from build123d import *

# Parameters (mm, degrees)
BOSS_EXTRUDE3_DEPTH = 30
CUT_EXTRUDE1_DEPTH  = 36.393360959
SKETCH12_W          = 4
SKETCH12_H          = 13
BOSS_EXTRUDE4_DEPTH = 30
BOSS_EXTRUDE9_REACH = 63.617
CUT_EXTRUDE3_DEPTH  = 55.655521025
CUT_EXTRUDE4_REACH  = 52.517


with BuildPart() as part:
    # Sketch7 → Boss-Extrude3 (new body)
    with BuildSketch(Plane.XY):
        Polygon((-1.7, -2), (-1.7, -15), (-5.7, -15), (-5.7, -2), (-9, -2), (-9, -15), (-13, -15), (-13, 1.250897452), align=None)
    extrude(amount=BOSS_EXTRUDE3_DEPTH)

    # Sketch11 → Cut-Extrude1 (cut, through all)
    with BuildSketch(Plane.ZY.offset(13)):
        Polygon((0, 1.250897452), (7.323081285, -15), (0, -15), align=None)
    extrude(amount=-CUT_EXTRUDE1_DEPTH, mode=Mode.SUBTRACT)

    # Sketch12 → Boss-Extrude4 (add, along a direction that is not the sketch's normal)
    with BuildSketch(Plane(origin=(0, -15, 0), x_dir=(-1, 0, 0), z_dir=(0, -1, 0))):
        with Locations((11, -13.823081285)):
            Rectangle(SKETCH12_W, SKETCH12_H)
        with Locations((3.7, -13.823081285)):
            Rectangle(SKETCH12_W, SKETCH12_H)
    extrude(amount=BOSS_EXTRUDE4_DEPTH, dir=(0, -0.9117077113862475, 0.4108394443074459))

    # Boss-Extrude9: up to this plane
    boss_extrude9_end = Plane(origin=(-1.7, -2, 30), z_dir=(-0.27647610983397475, -0.9610207909775272, 0))
    # Sketch18 → Boss-Extrude9 (add, up to the surface)
    with BuildSketch(Plane(origin=(0, -42.351231342, 0), x_dir=(-1, 0, 0), z_dir=(0, -1, 0)), mode=Mode.PRIVATE) as boss_extrude9_sk1:
        Polygon((1.7, -19.648264614), (13, -19.648264614), (13, -8.348264614), align=None)
    boss_extrude9_tool1 = split(extrude(boss_extrude9_sk1.sketch, amount=BOSS_EXTRUDE9_REACH, dir=(0, 0.911707711386, -0.410839444307), mode=Mode.PRIVATE), bisect_by=boss_extrude9_end, keep=Keep.BOTH, mode=Mode.PRIVATE)
    add(boss_extrude9_tool1.solids().sort_by_distance((-9.233333, -42.351231, 15.881598))[0])

    # Sketch19 → Cut-Extrude3 (cut, through all)
    with BuildSketch(Plane.ZY.offset(13)):
        Polygon((8.348264614, -42.351231342), (28.546690724, -33.249289946), (32.648264614, -42.351231342), align=None)
    extrude(amount=-CUT_EXTRUDE3_DEPTH, mode=Mode.SUBTRACT)

    # Cut-Extrude4: up to this plane
    cut_extrude4_end = Plane(origin=(-1.7, -2, 30), z_dir=(-0.27647610983397475, -0.9610207909775272, 0))
    # Sketch20 → Cut-Extrude4 (cut, up to the surface)
    with BuildSketch(Plane(origin=(0, -38.329779101, 17.272405344), x_dir=(-1, 0, 0), z_dir=(0, -0.9117077113862475, 0.4108394443074459)), mode=Mode.PRIVATE) as cut_extrude4_sk1:
        Polygon((13, 9.788379124), (10.050437985, 7.09924069), (13, 4.149152479), align=None)
    cut_extrude4_tool1 = split(extrude(cut_extrude4_sk1.sketch, amount=-CUT_EXTRUDE4_REACH, mode=Mode.PRIVATE), bisect_by=cut_extrude4_end, keep=Keep.BOTH, mode=Mode.PRIVATE)
    add(cut_extrude4_tool1.solids().sort_by_distance((-12.016813, -41.210691, 10.879276))[0], mode=Mode.SUBTRACT)

    # Mirror3: part across plane


with BuildPart() as part_1:
    add(part.part)
    add(part.part.mirror(Plane(origin=(-1.7, -2, 30), x_dir=(0, 0, 1), z_dir=(-0.27647610983397475, -0.9610207909775272, 0))))


solid = part_1.part
Read the model definition and answer for the solid it produces. Units are mm, in the model's axes. A direction names the side the tool comes from. Give positions to 0.01 mm unless a question says otherwise; leave off trailing zeros. Write each loop counter-clockwise with the first axis right and the second up, starting at its lowest first coordinate (ties: lowest second). Pieces come first, ordered by that corner, then holes. Notation, with made-up numbers: (36.25, 49.25) - (86.25, 49.25) arc R22 cw to (86.25, 87.25) - close; hole circle Ø4 at (27.25, 72.5). An arc over 180 degrees is marked (long way). Return JSON: item names as keys, results as strings.
Q1. A cutting plane is placed at A-A, the plane z = 27. Count the separate pieces of the cut face and the enclosed holes in it, and give its area (3 significant figures).
Reply:
{"separate pieces": "5", "enclosed holes": "0", "area": "311 mm²"}
Q2. Consider line 1 along Y through (x, z) = (-6.5, 24); line 2 along Y through (x, z) = (2.5, 18); line 3 along X through (y, z) = (24.5, 24.5). Determine where each line is inside the solid, lowest interval first. Write a range as [from, to].
Reply:
{"line 1": "[-2, 1.01], [4.09, 11.61]", "line 2": "[4.7, 12.22], [18.43, 25.96]", "line 3": "[1.58, 6.31], [10.2, 14.92]"}
Q3. A cutting plane is placed at C-C, the plane z = 15.5. Determine the outline of the cut face in (x, y) (3 decimals).
Reply:
{"outline": "(-13, -39.128) - (-4.396, -39.128) - (-1.7, -33.146) - (-1.7, -2) - (14.851, 24.384) - (15.746, 30.885) - (8.458, 35.457) - (-13, 1.251) - close; hole (-9, -33.146) - (-5.7, -33.146) - (-5.7, -2) - (-9, -2) - close; hole (-7.884, 1.879) - (-5.088, 0.126) - (11.462, 26.51) - (8.667, 28.263) - close"}
Q4. Given P1, Ø12, axis at x = 6, z = 3.5, coming from the +Y side; P2, Ø1.5, axis at x = 12, z = 13, coming from the +Y side; P3, Ø8, axis at x = 1.5, y = -28.5, coming from the +Z side, each flat-ended and moving along its own axis, determine where each tip first touches the part or whether it passes through.
Reply:
{"P1": "y = 31.32", "P2": "y = 35.18", "P3": "z = 27.49"}
Q5. For faces 1 (the face through (4.252, 16.357, 5.185)), 2 (the face through (-11, -15, 25)), 3 (the face through (3.264, 16.503, 9.717)), determine the directions among +Z, -Z, +X, -X, +Y, -Y from which every point of the face is accessible in a straight line to the end or side of a thin tool.
Reply:
{"face 1": "-Z, +X, -Y", "face 2": "+Z, +X, -X", "face 3": "+Z"}
Q6. A cutting plane is placed at D-D, the plane y = -11. Determine the outline of the cut face in (x, z).
Reply:
{"outline": "(-13, 0.41) - (-10.05, -2.83) - (-1.7, 5.52) - (-1.7, 30) - (-5.7, 30) - (-5.7, 5.52) - (-9, 5.52) - (-9, 30) - (-13, 30) - close"}
Q7. For a pull along X with two mould halves and no side action, classify faces 4 (the face through (-11.5, -20.12, 2.87)), 5 (the face through (-3.67, -24, 24.38)), 6 (the face through (-7, -2, 16)) as released by +X, released by -X, zero draft, split by the parting line, or undercut.
Reply:
{"face 4": "released by -X", "face 5": "zero draft", "face 6": "undercut"}
Q8. A cutting plane is placed at B-B, the plane y = -35. Determine the outline of the cut face in (x, z).
Reply:
{"outline": "(-13, 11.22) - (-10.05, 7.99) - (-1.7, 16.34) - (-1.7, 24.66) - (-5.7, 24.66) - (-5.7, 16.34) - (-9, 16.34) - (-9, 24.66) - (-13, 24.66) - close"}
